Job drawing, mm, ordinate dimensions from the low corner. One solid piece. A direction names the side the tool comes from. Give positions to 0.01 mm unless a question says otherwise; leave off trailing zeros. Write each loop counter-clockwise with the first axis right and the second up, starting at its lowest first coordinate (ties: lowest second). Pieces come first, ordered by that corner, then holes. Notation, with made-up numbers: M 11,57.25 L 37,57.25 A23 ccw 37,74.25 Z; hole C 61,83 d3. An arc over 180 degrees is marked long. Use CSV: the item, a comma, the result in double quotes. Start each with the question number.
Item 1: Cut at A-A (y = 12). List the corners of the cut face in (x, z).
Item 2: Pin check, flat tips, straight feed: pin 1 (1 mm diameter, centred on x = 55.5, z = 26, fed in from -Y); pin 2 (2 mm diameter, centred on y = 21, z = 9, fed in from -X); pin 3 (4.5 mm diameter, centred on x = 115.5, y = 23, fed in from -Z). Stop position of each tip, or through.
Item 3: Cut at B-B (x = 111.5). List the corners of the cut face in (y, z), then the cut area to 3 significant figures.
Item 4: Cut at C-C (z = 6). List the corners of the cut face in (x, y), then the cut area to 3 significant figures.
Item 5: Which spindle directions (+Z, -Z, +X, -X, +Y, -Y) get a long thin tool onto all of the face, cutting with end or side? Do the marked faces 1 and 2. Say none if no direction does.
Item 6: Cut at D-D (x = 10.5). List the corners of the cut face in (y, z).
Item 7: Drill centre lines: line 1 (X direction, y = 18.75, z = 30.5); line 2 (Z direction, x = 84, y = 9.75); line 3 (Y direction, x = 52.5, z = 27.5). Where is each one in solid material? Low to high. Write a range as [from, to].
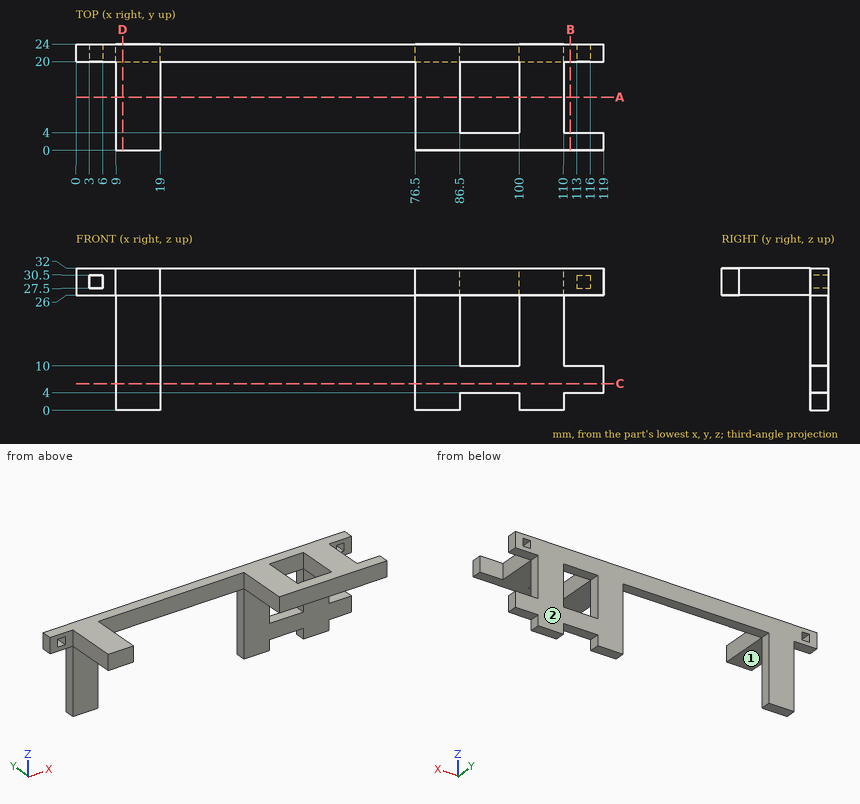
Worked answers:
1,outline,"M 9,26 L 19,26 L 19,32 L 9,32 Z; M 76.5,26 L 86.5,26 L 86.5,32 L 76.5,32 Z; M 100,26 L 110,26 L 110,32 L 100,32 Z"
2,pin 1,"stops at y = 20"
2,pin 2,"stops at x = 9"
2,pin 3,"stops at z = 4"
3,outline,"M 0,26 L 4,26 L 4,32 L 0,32 Z; M 20,4 L 24,4 L 24,10 L 20,10 Z; M 20,26 L 24,26 L 24,32 L 20,32 Z"
3,area,"72.0 mm^2"
4,outline,"M 9,20 L 19,20 L 19,24 L 9,24 Z; M 76.5,20 L 119,20 L 119,24 L 76.5,24 Z"
4,area,"210 mm^2"
5,face 1,"-Z, +X, -X, -Y"
5,face 2,"+Z, -Z, +X, -X, +Y"
6,outline,"M 0,26 L 20,26 L 20,0 L 24,0 L 24,32 L 0,32 Z"
7,line 1,"x = [9, 19], [76.5, 86.5], [100, 110]"
7,line 2,"z = [26, 32]"
7,line 3,"y = [20, 24]"
